Source: CAD feature listing. Evaluate the final solid. Frame: model axes, mm. A direction names the side the tool comes from. Give positions to 0.01 mm unless a question says otherwise; leave off trailing zeros. Order: outer loops, then holes, each group sorted by start corner. A loop starts at its lowest first (then second) coordinate and runs counter-clockwise, first axis right, second up.
from build123d import *

# Parameters (mm, degrees)
SKETCH3_W          = 34
SKETCH3_H          = 34
CUT_EXTRUDE1_DEPTH = 9


with BuildPart() as part:
    # Sketch1 → Revolve1 (revolve)
    with BuildSketch(Plane.XY):
        Polygon((0, 0), (0, 4.8), (0.2, 5), (4, 5), (4, 10.2), (9, 10.2), (9, 0), align=None)
    revolve(axis=Axis((9, 0, 0), (-1, 0, 0)))

    # Sketch2 → Cut-Revolve1 (revolve, cut)
    with BuildSketch(Plane.XY):
        Polygon((0, 0), (0, 3), (0.406, 2.594), (8.594, 2.594), (9, 3), (9, 0), align=None)
    revolve(axis=Axis((9, 0, 0), (-1, 0, 0)), mode=Mode.SUBTRACT)

    # Sketch3 → Cut-Extrude1 (cut)
    with BuildSketch(Plane(origin=(0, 0, 0), x_dir=(0, 0, -1), z_dir=(1, 0, 0))):
        Rectangle(SKETCH3_W, SKETCH3_H)
        Polygon((-9.814954576, 0), (-4.907477288, -8.5), (4.907477288, -8.5), (9.814954576, 0), (4.907477288, 8.5), (-4.907477288, 8.5), align=None, mode=Mode.SUBTRACT)
    extrude(amount=CUT_EXTRUDE1_DEPTH, mode=Mode.SUBTRACT)

    # Sketch4 → Cut-Revolve2 (revolve, cut)
    with BuildSketch(Plane(origin=(6.5, 0, 0), x_dir=(0, 0, -1), z_dir=(1, 0, 0))):
        Polygon((0, 8.5), (1.5, 8.5), (1.2295, 8.2295), (1.2295, 2.3645), (1.5, 2.094), (0, 2.094), align=None)
    revolve(axis=Axis((6.5, 2.094, 0), (0, 1, 0)), mode=Mode.SUBTRACT)

    # Sketch5 → Cut-Revolve3 (revolve, cut)
    with BuildSketch(Plane(origin=(6.5, 0, 0), x_dir=(0, 0, -1), z_dir=(1, 0, 0))):
        Polygon((7.361215932, -4.25), (6.611215932, -5.549038106), (6.51220606, -5.179528234), (1.432967067, -2.247028234), (1.063457196, -2.346038106), (1.813457196, -1.047), align=None)
    revolve(axis=Axis((6.5, -1.047, -1.813457196), (0, -0.5, -0.866025404)), mode=Mode.SUBTRACT)


solid = part.part
1) First-contact query: pin 1 Ø2 at (x, z) = (4.5, -6.5) entering from +Y; pin 2 Ø1.5 at (x, y) = (2, -2) entering from -Z. Flat tips, straight axial feed; report the tip coordinate or a pass-through.
Checks:
pin 1: stops at y = 7.47
pin 2: stops at z = -4.84
2) Section query B-B on x = 6.5. Output: boundary loops of the cut face in (y, z), and give its area (3 significant figures).
Checks:
outline: (-8.5, -4.91) - (-5.55, -6.61) - (-5.18, -6.51) - (-2.25, -1.43) - (-2.32, -1.16) arc R2.59 cw to (2.16, 1.43) - (2.36, 1.23) - (8.23, 1.23) - (8.5, 1.5) - (8.5, 4.91) - (0, 9.81) - (-8.5, 4.91) - close; (-3.05, -7.74) - (-2.95, -8.11) - (0, -9.81) - (8.5, -4.91) - (8.5, -1.5) - (8.23, -1.23) - (2.36, -1.23) - (2.16, -1.43) arc R2.59 cw to (0.16, -2.59) - (-0.12, -2.66) - close
area: 199 mm2
3) Section query C-C on y = 5.75. Output: boundary loops of the cut face in (x, z).
Checks:
outline: (4, -6.5) - (9, -6.5) - (9, 6.5) - (4, 6.5) - close; hole circle Ø2.46 at (6.5, 0)
4) Section query D-D on x = 1.75. Output: boundary loops of the cut face in (y, z), and give its area (3 significant figures).
Checks:
outline: circle Ø10 at (0, 0); hole circle Ø5.19 at (0, 0)
area: 57.4 mm2
5) Pull-direction query (Y, two-part tool) for faces 4 (the face through (4.557, -0.562, 2.532)), 5 (the face through (2.13, -1.08, 4.88)), 6 (the face through (6.465, 4.191, -7.396)); classes: +Y half, -Y half, draft (parallel to the pull), parting line (faces both ways), or undercut.
Checks:
face 4: undercut
face 5: parting line
face 6: +Y half
6) Reachability of faces 1 (the face through (4, -4, 4)), 2 (the face through (6.465, -4.191, 7.396)), 3 (the face through (7.7, 5.26, 0.27)) from +Z, -Z, +X, -X, +Y, -Y: full face, straight path, thin tool, end or side. Return the list, or none.
Checks:
face 1: -X
face 2: +Z, +X, -X, -Y
face 3: +Y
7) Section query A-A on z = 0. Output: boundary loops of the cut face in (x, y), and give its area (3 significant figures).
Checks:
outline: (0, -4.8) - (0.2, -5) - (4, -5) - (4, -8.5) - (9, -8.5) - (9, -3) - (8.59, -2.59) - (0.41, -2.59) - (0, -3) - close; (0, 3) - (0.41, 2.59) - (5.27, 2.59) - (5.27, 8.23) - (5, 8.5) - (4, 8.5) - (4, 5) - (0.2, 5) - (0, 4.8) - close; (7.73, 2.59) - (8.59, 2.59) - (9, 3) - (9, 8.5) - (8, 8.5) - (7.73, 8.23) - close
area: 63.3 mm2
8) Ray query, L1, parallel to X at y = 3.9, z = 0; L2, parallel to X at y = 6, z = 0; L3, parallel to Y at x = 4.75, z = 0. Return the intervals inside material, ascending.
Checks:
L1: x = 0 to 5.27, 7.73 to 9
L2: x = 4 to 5.27, 7.73 to 9
L3: y = -8.5 to -2.59, 2.59 to 8.5
